```python
from build123d import *

# Parameters (mm, degrees)
SKETCH_1_W          = 14
SKETCH_1_H          = 14
EXTRUDE_2_DEPTH     = 3
EXTRUDE_4_DEPTH     = 3
EXTRUDE_5_DEPTH     = 3
SKETCH_4_R          = 0.8
CUT_EXTRUDE_1_DEPTH = 3
SKETCH_5_R          = 7
EXTRUDE_6_DEPTH     = 8
SKETCH_6_R          = 6.4
CUT_EXTRUDE_2_DEPTH = 7


with BuildPart() as part:
    # 草图1 → 凸台-拉伸2 (new body)
    with BuildSketch(Plane(origin=(0, 0, 0), x_dir=(1, 0, 0), z_dir=(0, 1, 0))):
        Rectangle(SKETCH_1_W, SKETCH_1_H)
    extrude(amount=EXTRUDE_2_DEPTH)

    # 草图2 → 凸台-拉伸4 (add)
    with BuildSketch(Plane(origin=(0, 3, 0), x_dir=(1, 0, 0), z_dir=(0, 1, 0))):
        Polygon((-7, 0), (-7, 2), (-9, 2), (-9, 0), (-9, -2), (-7, -2), align=None)
        Polygon((7, 0), (7, 2), (9, 2), (9, 0), (9, -2), (7, -2), align=None)
    extrude(amount=-EXTRUDE_4_DEPTH)

    # 草图3 → 凸台-拉伸5 (add)
    with BuildSketch(Plane(origin=(0, 3, 0), x_dir=(1, 0, 0), z_dir=(0, 1, 0))):
        with BuildLine():
            Line((-9, 2), (-9, -2))
            ThreePointArc((-9, -2), (-11, 0), (-9, 2))
        make_face()
        with BuildLine():
            Line((9, 2), (9, -2))
            ThreePointArc((9, -2), (11, 0), (9, 2))
        make_face()
    extrude(amount=-EXTRUDE_5_DEPTH)

    # 草图4 → 切除-拉伸1 (cut)
    with BuildSketch(Plane(origin=(0, 3, 0), x_dir=(1, 0, 0), z_dir=(0, 1, 0))):
        with Locations((-9, 0)):
            Circle(SKETCH_4_R)
        with Locations((9, 0)):
            Circle(SKETCH_4_R)
    extrude(amount=-CUT_EXTRUDE_1_DEPTH, mode=Mode.SUBTRACT)

    # 草图5 → 凸台-拉伸6 (add)
    with BuildSketch(Plane(origin=(0, 3, 0), x_dir=(1, 0, 0), z_dir=(0, 1, 0))):
        Circle(SKETCH_5_R)
    extrude(amount=EXTRUDE_6_DEPTH)

    # 草图6 → 切除-拉伸2 (cut)
    with BuildSketch(Plane(origin=(0, 11, 0), x_dir=(1, 0, 0), z_dir=(0, 1, 0))):
        Circle(SKETCH_6_R)
    extrude(amount=-CUT_EXTRUDE_2_DEPTH, mode=Mode.SUBTRACT)


solid = part.part
```
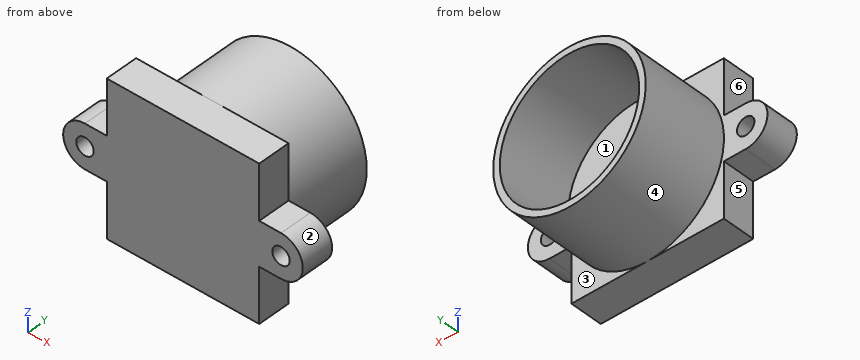
CAD build for the part. Positions are in the model's coordinates, mm. Face numbers are marked on the shaded views. A direction names the side the tool comes from. Round coordinates to 2 decimals unless told otherwise and drop trailing zeros. Loops run counter-clockwise (first coordinate to the right, second up) from the corner with the lowest first, then second, coordinate; pieces in that order, holes last. Notation, with made-up numbers: M 62.25,-15.75 L 96.25,-15.75 A16 cw 96.25,6.25 Z; hole C 81.5,-37 d2. An arc over 180 degrees is marked long. Return JSON: item names as keys, results as strings. Group by question number.
(1) Drop flat-ended pins along their axis: P1, Ø1, axis at y = 7, z = 2, coming from the -X side; P2, Ø8, axis at x = 0.5, z = 3, coming from the +Y side; P3, Ø1, axis at x = 8, y = 2, coming from the -Z side; P4, Ø2.5, axis at y = 1, z = 3.5, coming from the -X side. Give the stop position or say it passes through.
(2) Wall check: probe 1 along X at (y, z) = (1.35, 0); probe 2 along Z at (x, y) = (-9, 1.35); probe 3 along X at (y, z) = (5.75, -0.25). Give the ranges that are in metal, low to high. Write a range as [from, to].
(3) Mould opens along Z. For the marked faces 1, 2 and 3 say: +Z half, -Z half, draft (parallel to the pull), parting line (faces both ways), or undercut.
(4) Saw through at B-B, the plane y = 10.5. List the corners of the cut face in (x, z).
(5) Saw through at C-C, the plane x = -5. List the corners of the cut face in (y, z) (3 decimals).
(6) Tool access for the marked faces 4, 5 and 6: list every direction of +Z, -Z, +X, -X, +Y, -Y with a clear straight run to the whole face (end or side of a thin tool).
(7) Saw through at A-A, the plane z = 0. List the corners of the cut face in (x, y).
(8) Saw through at D-D, the plane z = 3.5. List the corners of the cut face in (x, y).
Answer list:
{
 "1": {"P1": "x = -6.84", "P2": "y = 11", "P3": "z = -2", "P4": "x = -7"},
 "2": {"probe 1": "[-11, -9.8], [-8.2, 8.2], [9.8, 11]", "probe 2": "[-2, -0.8], [0.8, 2]", "probe 3": "[-7, -6.4], [6.4, 7]"},
 "3": {"face 1": "undercut", "face 2": "parting line", "face 3": "draft"},
 "4": {"outline": "C 0,0 d14; hole C 0,0 d12.8"},
 "5": {"outline": "M 0,-7 L 3,-7 L 3,-4.899 L 11,-4.899 L 11,-3.995 L 4,-3.995 L 4,3.995 L 11,3.995 L 11,4.899 L 3,4.899 L 3,7 L 0,7 Z"},
 "6": {"face 4": "+Y", "face 5": "-Z, -X, +Y, -Y", "face 6": "+Z, -X, +Y, -Y"},
 "7": {"outline": "M -11,0 L -9.8,0 L -9.8,3 L -11,3 Z; M -8.2,0 L 8.2,0 L 8.2,3 L 7,3 L 7,11 L 6.4,11 L 6.4,4 L -6.4,4 L -6.4,11 L -7,11 L -7,3 L -8.2,3 Z; M 9.8,0 L 11,0 L 11,3 L 9.8,3 Z"},
 "8": {"outline": "M -7,0 L 7,0 L 7,3 L 6.06,3 L 6.06,11 L 5.36,11 L 5.36,4 L -5.36,4 L -5.36,11 L -6.06,11 L -6.06,3 L -7,3 Z"}
}
